Design review of the part shown in the three views and the two pictorial views. Dimensions are in mm from the part's minimum x, y and z. A direction names the side the tool comes from. Coordinates: 2 decimals unless noted, no trailing zeros. Loops run counter-clockwise (first coordinate to the right, second up) from the corner with the lowest first, then second, coordinate; pieces in that order, holes last.
Q1. Add section A-A on x = 75. Give the boundary of the cut face in (y, z), and give its area (3 significant figures).
Q2. Add section D-D on y = 12. Give the boundary of the cut face in (x, z), and give its area (3 significant figures).
Q3. For P1, Ø5, axis at x = 108.5, z = 127.5, coming from the +Y side; P2, Ø1.5, axis at y = 9, z = 127, coming from the +X side; P3, Ø5, axis at x = 13, z = 73, coming from the +Y side; P4, Ø2, axis at y = 11.5, z = 93, coming from the -X side, all flat-tipped, find the tip position at first contact; note any pin that passes through.
Q4. Machinability: for the marked faces 4 and 5, which of the approach directions +Z, -Z, +X, -X, +Y, -Y give a long, thin tool a straight path to every point of the face, cutting with its end or side? Answer none if there is none.
Q5. Wall thickness on probe 1 along Z at (x, y) = (75, 11.1); probe 2 along Z at (x, y) = (107.5, 1.5) (1 decimal); probe 3 along Y at (x, z) = (94, 73): over which ranges is each line inside the solid? List them lowest first.
Q6. Add section C-C on x = 106.25. Give the boundary of the cut face in (y, z).
Q7. Draft analysis for pull direction Z (two halves, no side actions). For the marked faces 1, 2 and 3, state which applies: released by +Z, released by -Z, zero draft, split by the parting line, or undercut.
Q8. Add section B-B on z = 75. Give the boundary of the cut face in (x, y).
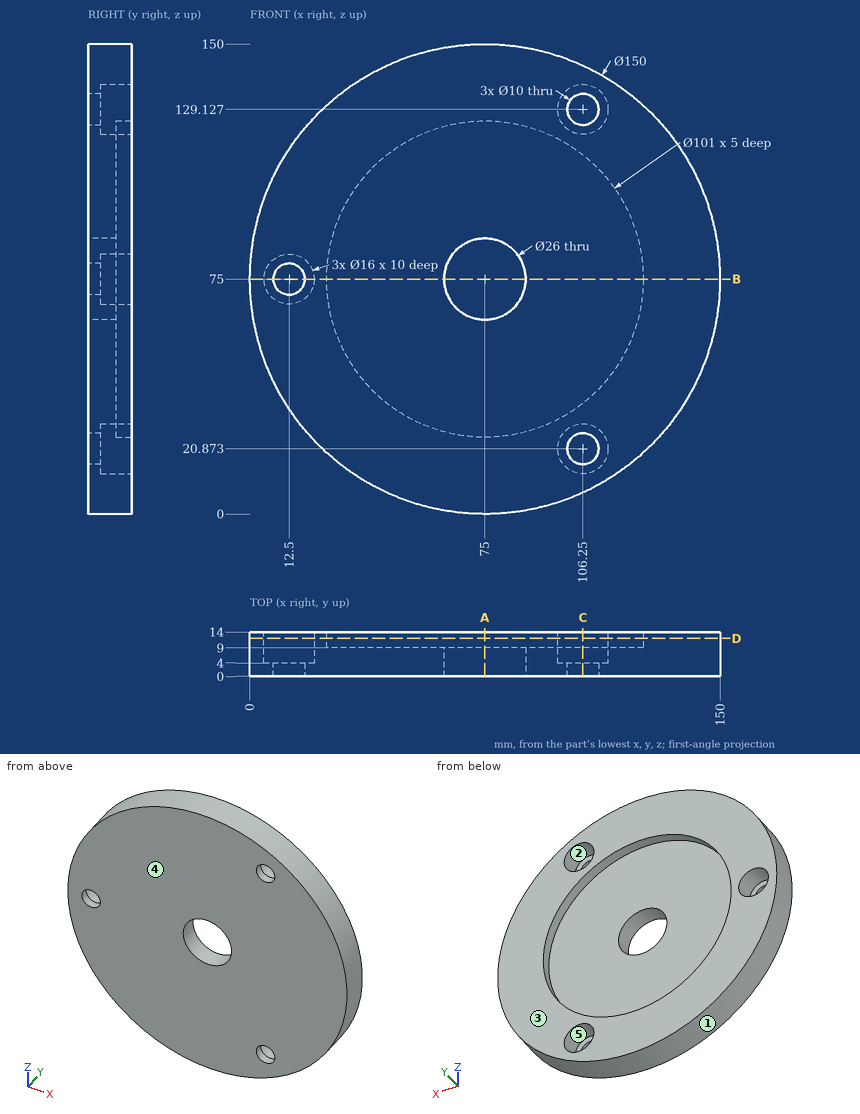
Entries:
1. outline: (0, 0) - (14, 0) - (14, 24.5) - (9, 24.5) - (9, 62) - (0, 62) - close; (0, 88) - (9, 88) - (9, 125.5) - (14, 125.5) - (14, 150) - (0, 150) - close
1. area: 1,360 mm2
2. outline: circle Ø150 at (75, 75); hole circle Ø16 at (12.5, 75); hole circle Ø101 at (75, 75); hole circle Ø16 at (106.25, 20.87); hole circle Ø16 at (106.25, 129.13)
2. area: 9,060 mm2
3. P1: stops at y = 4
3. P2: stops at x = 129.76
3. P3: passes through
3. P4: stops at x = 1.95
4. face 4: +Z, -Z, +X, -X, -Y
4. face 5: +Y
5. probe 1: z = 0 to 24.5, 125.5 to 150
5. probe 2: z = 7.4 to 16, 25.7 to 124.3, 134 to 142.6
5. probe 3: y = 0 to 9
6. outline: (0, 6.82) - (14, 6.82) - (14, 12.87) - (4, 12.87) - (4, 15.87) - (0, 15.87) - close; (0, 25.87) - (4, 25.87) - (4, 28.87) - (14, 28.87) - (14, 35.33) - (9, 35.33) - (9, 114.67) - (14, 114.67) - (14, 121.13) - (4, 121.13) - (4, 124.13) - (0, 124.13) - close; (0, 134.13) - (4, 134.13) - (4, 137.13) - (14, 137.13) - (14, 143.18) - (0, 143.18) - close
7. face 1: split by the parting line
7. face 2: undercut
7. face 3: zero draft
8. outline: (0, 0) - (7.5, 0) - (7.5, 4) - (4.5, 4) - (4.5, 14) - (0, 14) - close; (17.5, 0) - (62, 0) - (62, 9) - (24.5, 9) - (24.5, 14) - (20.5, 14) - (20.5, 4) - (17.5, 4) - close; (88, 0) - (150, 0) - (150, 14) - (125.5, 14) - (125.5, 9) - (88, 9) - close
